```python
from build123d import *

# Parameters (mm, degrees)
F0_W     = 5
F0_H     = 30
F1_DEPTH = 16
F2_R     = 5
F3_R     = 2.49999


# Not quite as in the source:
# - a fillet or chamfer is up to 0.001 mm smaller than in the source, because OpenCascade refuses the exact size
# - a feature names something its author has since deleted; it is built from what else it names


with BuildPart() as f1:
    # F0 (on Top) → F1 (new body)
    with BuildSketch(Plane.XY):
        with Locations((-13, -119.1857503612)):
            Rectangle(F0_W, F0_H)
        Polygon((-15.5, -99.1857503612), (-15.5, -104.1857503612), (-10.5, -104.1857503612), (-5, -104.1857503612), (0, -104.1857503612), (0, -99.1857503612), align=None)
        Polygon((0, -104.1857503612), (-5, -104.1857503612), (-5, -134.1857503612), (0, -134.1857503612), (0, -129.1857503612), align=None)
        Polygon((22.0267780379, -99.1857503612), (0, -99.1857503612), (0, -104.1857503612), (17.5957249839, -104.1857503612), (20.6230915981, -129.1857503612), (0, -129.1857503612), (0, -134.1857503612), (25.6551948256, -134.1857503612), (46.11123117, -131.7086335017), (44.067551515, -114.8319225227), (39.1038129917, -115.4330047742), (40.5464103953, -127.3459772299), (25.6551948256, -129.1492239844), align=None)
    extrude(amount=F1_DEPTH)

    # F2
    f2_edges = [f1.edges().sort_by_distance(p)[0] for p in [
        (-15.5, -99.18575, 8),
        (0, -104.18575, 8),
        (17.595725, -104.18575, 8),
        (20.623092, -129.18575, 8),
        (0, -129.18575, 8),
        (-5, -134.18575, 8),
        (22.026778, -99.18575, 8),
        (25.655195, -134.18575, 8),
        (46.111231, -131.708634, 8),
    ]]
    fillet(f2_edges, radius=F2_R)

    # F3 (radius 2.5 in the source; OpenCascade refuses exactly that, so slightly less here)
    f3_edges = [f1.edges().sort_by_distance(p)[0] for p in [
        (44.067552, -114.831923, 8),
        (39.103813, -115.433005, 8),
        (-15.5, -134.18575, 8),
        (-10.5, -134.18575, 8),
        (-10.5, -104.18575, 8),
        (-5, -104.18575, 8),
        (25.655195, -129.149224, 8),
        (40.54641, -127.345977, 8),
    ]]
    fillet(f3_edges, radius=F3_R)


solid = f1.part
```
Could you check a few things on this model? Use its own coordinates, in mm. A direction names the side the tool comes from. Coordinates: 2 decimals unless noted, no trailing zeros. Loops run counter-clockwise (first coordinate to the right, second up) from the corner with the lowest first, then second, coordinate; pieces in that order, holes last.
1) Imagine slicing it at C-C (y = -112). List the corners of the cut face in (x, z) for me, and give its area (3 significant figures).
Reported:
outline: (-15.5, 0) - (-10.5, 0) - (-10.5, 16) - (-15.5, 16) - close; (-5, 0) - (0, 0) - (0, 16) - (-5, 16) - close; (18.54, 0) - (23.58, 0) - (23.58, 16) - (18.54, 16) - close
area: 241 mm2
2) Which directions (+Z, -Z, +X, -X, +Y, -Y) give clear straight access to the entire face, cutting with the end or side of a thin tool? Please do faces 1 (the face through (1.426, -105.689, 8.112)), 2 (the face through (23.977, -115.288, 7.888)), 3 (the face through (4, -99.186, 8)), 4 (the face through (-5, -118, 8)).
Reported:
face 1: +Z, -Z
face 2: +Z, -Z, +Y
face 3: +Z, -Z, +X, -X, +Y
face 4: +Z, -Z, -Y
3) Thinking about a two-plate mould opening in X: for faces 5 (the face through (18.76, -127.46, 8.11)), 6 (the face through (21, -120, 16)), 7 (the face through (44.45, -130.47, 8.11)), which applies, released by +X, released by -X, zero draft, split by the parting line, or undercut?
Reported:
face 5: undercut
face 6: zero draft
face 7: released by +X
4) Imagine slicing it at B-B (x = 10). List the corners of the cut face in (y, z) for me.
Reported:
outline: (-134.19, 0) - (-129.19, 0) - (-129.19, 16) - (-134.19, 16) - close; (-104.19, 0) - (-99.19, 0) - (-99.19, 16) - (-104.19, 16) - close
5) Please list where these lines run through material, in increasing order: line 1 along Y through (x, z) = (5, 10); line 2 along X through (y, z) = (-112, 13); line 3 along X through (y, z) = (-117.5, 11.75).
Reported:
line 1: y = -134.19 to -129.19, -104.19 to -99.19
line 2: x = -15.5 to -10.5, -5 to 0, 18.54 to 23.58
line 3: x = -15.5 to -10.5, -5 to 0, 19.21 to 24.24, 39.39 to 44.39
6) Imagine slicing it at D-D (y = -108). List the corners of the cut face in (x, z) for me, and give its area (3 significant figures).
Reported:
outline: (-15.5, 0) - (-10.5, 0) - (-10.5, 16) - (-15.5, 16) - close; (-5, 0) - (0.14, 0) - (0.14, 16) - (-5, 16) - close; (18.02, 0) - (23.09, 0) - (23.09, 16) - (18.02, 16) - close
area: 243 mm2
7) Will these pins go through, and if not, where does the flat tip stop? pin 1 Ø8 at (x, z) = (36, 9) entering from -Y; pin 2 Ø6 at (x, z) = (30.5, 14) entering from -Y; pin 3 Ø4.5 at (y, z) = (-115, 4.5) entering from +X.
Reported:
pin 1: stops at y = -133.42
pin 2: stops at y = -133.96
pin 3: stops at x = 44.36
